Autodesk Inventor part; units mm, degrees
ref_plane "YZ Plane" through (0, 0, 0) normal (1, 0, 0) x (0, 1, 0)
ref_plane "XZ Plane" through (0, 0, 0) normal (0, 1, 0) x (-1, 0, 0)
ref_plane "XY Plane" through (0, 0, 0) normal (0, 0, 1) x (1, 0, 0)
sketch "草圖1" plane through (0, 0, 0) normal (0, 0, 1) x (1, 0, 0)
  arc A0 (-17.5, 0) -> (17.5, 0) centre (0, 0) ccw
  arc A1 (-20, 0) -> (20, 0) centre (0, 0) ccw
  line L0 (-20, 0) -> (-17.5, 0)
  line L1 (20, 0) -> (17.5, 0)
  line L2 (-35, 0) -> (35, 0)
  line L3 (-25, 0) -> (25, 0)
  line L4 (25, -75) -> (-25, -75)
  line L5 (-25, -75) -> (-25, 0)
  line L6 (-25, 0) -> (25, 0)
  line L7 (25, 0) -> (25, -75)
  line L8 (25, -75) -> (-25, 0) construction
  line L9 (-25, -75) -> (25, 0) construction
  line L10 (0, -90) -> (0, 15)
  point P0 (17.5, 0)
  point P1 (20, 0)
  point P2 (20, 0)
  point P3 (0, -37.5)
  dimension "d0" = 17.5
  dimension "d16" = 50
  dimension "d17" = 75
  dimension "d22" = 20
extrude "擠出1" add sketch "草圖1" along normal mid plane 20 contours L2 L10 A0 | A0 L10 A1 L0 | L10 L2 A0 | A0 L1 A1 L10
extrude "擠出2" add sketch "草圖1" along normal mid plane 5
sketch "草圖2" plane through (0, 0, 0) normal (1, 0, 0) x (0, 1, 0)
  line L0 (-10, -10) -> (-5, 10)
  line L1 (0, -2.5) -> (0, -10)
  line L2 (0, 10) -> (0, 2.5)
  line L3 (-20, -10) -> (0, -10)
  line L4 (0, 10) -> (-20, 10)
  point P0 (0, 0)
  dimension "d18" = 10
  dimension "d19" = 5
sketch "草圖3" plane through (0, 0, -10) normal (0, 0, -1) x (-1, 0, 0)
  arc A0 (-17.5, 0) -> (17.5, 0) centre (0, 0) ccw
  line L0 (25, 0) -> (-25, 0)
sweep "掃掠1" cut profiles "草圖3" path "草圖2" path curves L0
Here's how the part is built. I have some questions about the finished solid (model axes, mm). A direction names the side the tool comes from. Coordinates: 2 decimals unless noted, no trailing zeros. Write each loop counter-clockwise with the first axis right and the second up, starting at its lowest first coordinate (ties: lowest second). Pieces come first, ordered by that corner, then holes.
1) If we section it at A-A (y = -37): List the corners of the cut face in (x, z) for me.
Filled in:
outline: (-25, -2.5) - (25, -2.5) - (25, 2.5) - (-25, 2.5) - close
2) I'm going to push flat-ended pins straight in: pin 1 (8 mm diameter, centred on x = -6.5, z = -6.5, fed in from +Y); pin 2 (3 mm diameter, centred on y = -13.5, z = 5.5, fed in from -X); pin 3 (1 mm diameter, centred on y = -18.5, z = 6, fed in from +X); pin 4 (4 mm diameter, centred on x = -19, z = 1, fed in from +Y). Where does each tip first touch, or does it pass through?
Filled in:
pin 1: stops at y = -12.96
pin 2: stops at x = -16
pin 3: stops at x = 8.72
pin 4: stops at y = 0
3) If we section it at B-B (x = -19): List the corners of the cut face in (y, z) for me (3 decimals).
Filled in:
outline: (-75, -2.5) - (-6.245, -2.5) - (-6.245, -10) - (0, -10) - (0, 10) - (-6.245, 10) - (-6.245, 2.5) - (-75, 2.5) - close
4) Which directions (+Z, -Z, +X, -X, +Y, -Y) give clear straight access to the entire face, cutting with the end or side of a thin tool? Please do faces 1 (the face through (0, -20, -6)), 2 (the face through (25, -37, 0)), 3 (the face through (0, -20, 6)).
Filled in:
face 1: -Z, -Y
face 2: +Z, -Z, +X, +Y, -Y
face 3: +Z, -Y
5) If I drill on line 1 (Z direction, x = 3.5, y = -27.5); line 2 (X direction, y = -8.5, z = -8.75); line 3 (X direction, y = -14, z = 9), over which ranges is the centre line in solid material (lowest first)?
Filled in:
line 1: z = -2.5 to 2.5
line 2: x = -18.1 to -15.12, 15.12 to 18.1
line 3: x = -14.28 to 14.28
